Source: three-view drawing plus pictorial views. Frame: mm from the lowest corner of the part. Give positions to 0.01 mm unless a question says otherwise; leave off trailing zeros. Order: outer loops, then holes, each group sorted by start corner. A loop starts at its lowest first (then second) coordinate and runs counter-clockwise, first axis right, second up. Notation, with made-up numbers: M 7.5,-1.75 L 11.5,-1.75 A7 ccw 11.5,5.25 Z; hole C -12,17 d9. An arc over 180 degrees is marked long. Use CSV: the item, a comma, the result in double quotes.
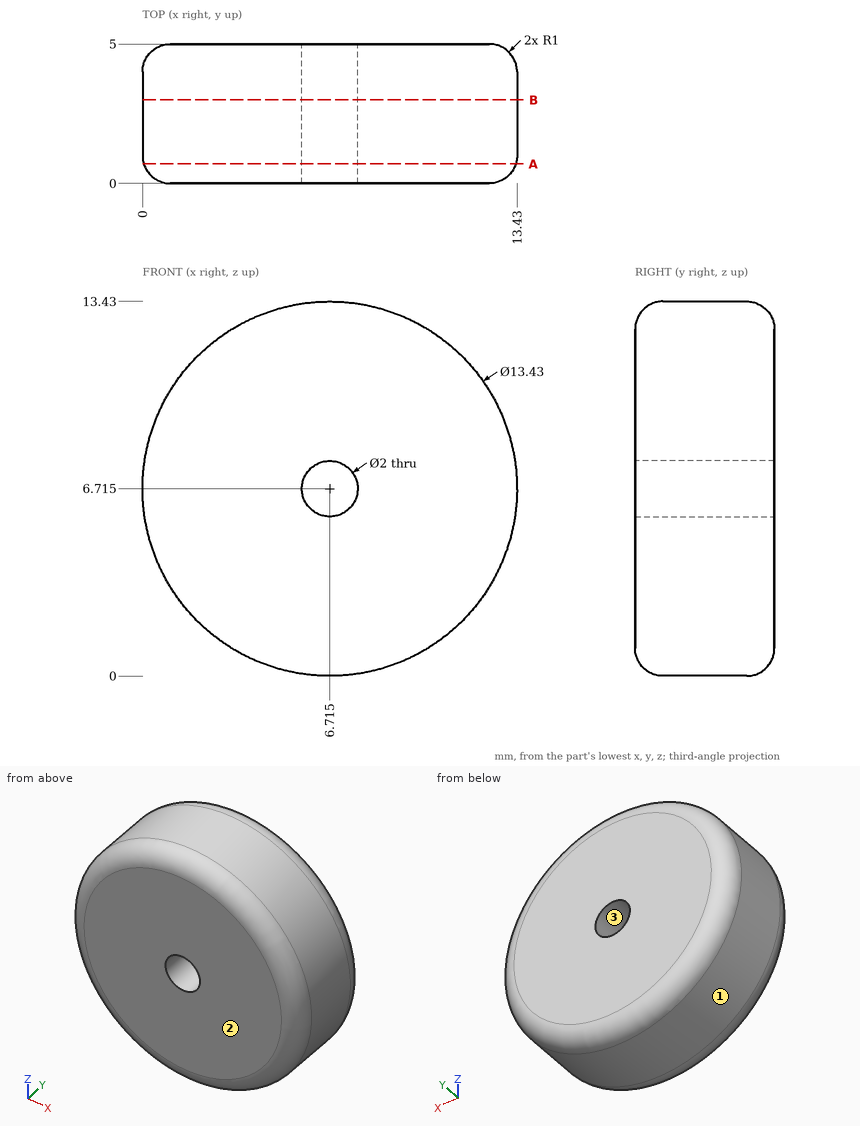
1. Section B-B, the plane y = 3. Return the cut outline in (x, z) (3 decimals).
Answer:
outline,"C 6.715,6.715 d13.43; hole C 6.715,6.715 d2"
2. Section A-A, the plane y = 0.7. Return the cut outline in (x, z) (3 decimals), plus the area to 3 significant figures.
Answer:
outline,"C 6.715,6.715 d13.338; hole C 6.715,6.715 d2"
area,"137 mm2"
3. Pin query (flat end, axial travel): pin 1 Ø1 at (x, y) = (3.5, 1.5) entering from +Z; pin 2 Ø1.8 at (x, z) = (6.715, 6.715) entering from +Y; pin 3 Ø1 at (y, z) = (3, 12) entering from -X. Return the tip coordinate at first contact, or that it passes through.
Answer:
pin 1,"z = 12.86"
pin 2,"through"
pin 3,"x = 2"
4. Pull-direction query (X, two-part tool) for the marked faces 1, 2 and 3; classes: +X half, -X half, draft (parallel to the pull), parting line (faces both ways), or undercut.
Answer:
face 1,"parting line"
face 2,"draft"
face 3,"undercut"
5. Line query: line 1 (X direction, y = 2.5, z = 6.75); line 2 (X direction, y = 0.55, z = 7); line 3 (X direction, y = 3.7, z = 1.75). Output: solid intervals per line, ascending.
Answer:
line 1,"0 to 5.72, 7.71 to 13.43"
line 2,"0.11 to 5.76, 7.67 to 13.32"
line 3,"2.19 to 11.24"
